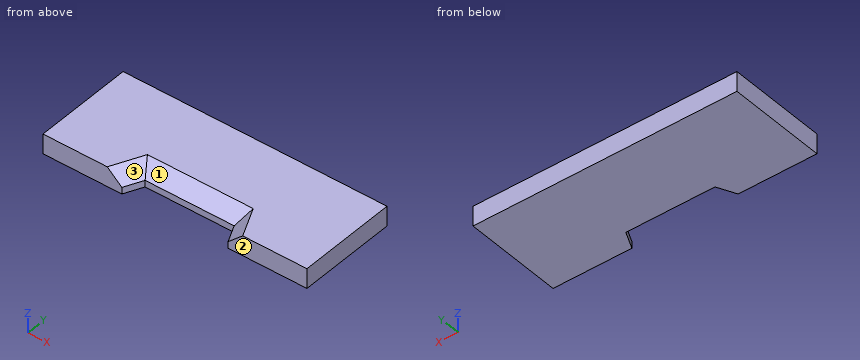
from build123d import *

# Parameters (mm, degrees)
F1_DEPTH = 3
F2_SIZE  = 2


# Not quite as in the source:
# - a feature names something its author has since deleted; it is built from what else it names


with BuildPart() as f1:
    # F0 (on Top) → F1 (new body)
    with BuildSketch(Plane.XY):
        Polygon((8.05, -7.5), (20, -7.5), (20, 7.5), (-20, 7.5), (-20, -7.5), (-8.05, -7.5), (-6.75, -4.75), (0, -4.75), (6.75, -4.75), align=None)
    extrude(amount=F1_DEPTH)

    # F2
    f2_edges = [f1.edges().sort_by_distance(p)[0] for p in [
        (-7.4, -6.125, 3),
        (0, -4.75, 3),
        (7.4, -6.125, 3),
    ]]
    chamfer(f2_edges, length=F2_SIZE)


solid = f1.part
Here's how the part is built. I have some questions about the finished solid (model axes, mm). Face numbers are marked on the shaded views. Coordinates: 2 decimals unless noted, no trailing zeros. Loops run counter-clockwise (first coordinate to the right, second up) from the corner with the lowest first, then second, coordinate; pieces in that order, holes last. Notation, with made-up numbers: (57.25, 40.5) -> (105.25, 40.5) arc R9 ccw to (105.25, 56.5) -> close; hole circle Ø8 at (-35, -40). An arc over 180 degrees is marked (long way). Use one line per item in the form item = value. Start each with the question number.
(1) If we section it at A-A (z = 0.6): Please give me the cut outline in (x, y), then the cut area to 3 significant figures.
(2) Please list where these lines run through material, in increasing order: line 1 along X through (y, z) = (-4, 2); line 2 along X through (y, z) = (-4.25, 2); line 3 along Y through (x, z) = (8, 2.8).
(3) Will these pins go through, and if not, where does the flat tip stop? pin 1 (1.1 mm diameter, centred on x = 2.5, z = 0.5, fed in from -Y); pin 2 (3 mm diameter, centred on x = 9.5, y = 3, fed in from -Z).
(4) If we section it at B-B (y = -4): Please give me the cut outline in (x, z), then the cut area to 3 significant figures.
(5) We'd pull the mould along X, two halves only. Please class the marked faces 1, 2 and 3: pulls with the +X half, pulls with the -X half, needs draft (parallel to the pull), parting line crosses it, or undercut.
(6) If we section it at C-C (x = 4.5): Please give me the cut outline in (y, z).
Verdict:
q1.outline = (-20, -7.5) -> (-8.05, -7.5) -> (-6.75, -4.75) -> (6.75, -4.75) -> (8.05, -7.5) -> (20, -7.5) -> (20, 7.5) -> (-20, 7.5) -> close
q1.area = 559 mm²
q2.line_1 = -20 to -7.5, 7.5 to 20
q2.line_2 = -20 to -7.62, 7.62 to 20
q2.line_3 = -3.18 to 7.5
q3.pin_1 = -4.75
q3.pin_2 = 0
q4.outline = (-20, 0) -> (20, 0) -> (20, 3) -> (8.61, 3) -> (7.23, 1.75) -> (-7.23, 1.75) -> (-8.61, 3) -> (-20, 3) -> close
q4.area = 100 mm²
q5.face_1 = undercut
q5.face_2 = needs draft
q5.face_3 = undercut
q6.outline = (-4.75, 0) -> (7.5, 0) -> (7.5, 3) -> (-2.75, 3) -> (-4.75, 1) -> close
